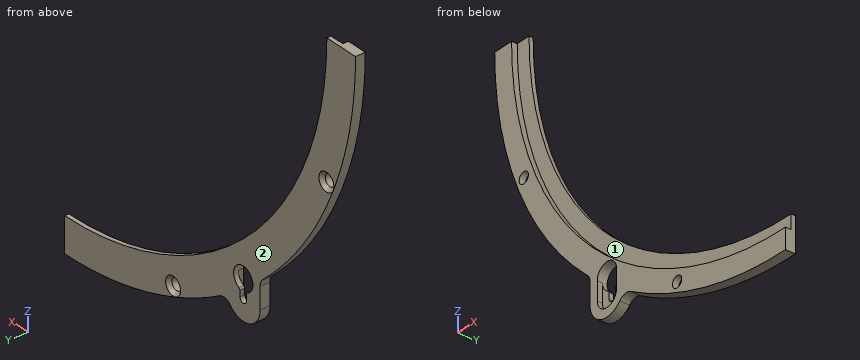
```python
from build123d import *

# Parameters (mm, degrees)
CUT_EXTRUDE2_DEPTH                   = 25.4
F_6_0_204_DIAMETER_HOLE1_D           = 5.499999922
F_6_0_204_DIAMETER_HOLE1_CSINK_D     = 8.89
F_6_0_204_DIAMETER_HOLE1_CSINK_ANGLE = 90
BOSS_EXTRUDE2_REACH                  = 245.998
CUT_EXTRUDE3_DEPTH                   = 244.998078886
CUT_EXTRUDE4_DEPTH                   = 2.5
FILLET1_R                            = 5
FILLET3_R                            = 1


with BuildPart() as part:
    # Sketch1 → Revolve1 (revolve)
    with BuildSketch(Plane.XY, mode=Mode.PRIVATE) as revolve1_sk:
        Polygon((-162.5, 0), (-162.5, 2.75), (-155.5, 2.75), (-155.5, 4.75), (-172.5, 4.75), (-172.5, 0), align=None)
    revolve(revolve1_sk.sketch.rotate(Axis((0, 0, 0), (0, 1, 0)), 270), axis=Axis((0, 0, 0), (0, 1, 0)))

    # Sketch5 → Cut-Extrude2 (cut, symmetric)
    with BuildSketch(Plane(origin=(0, 0, 0), x_dir=(1, 0, 0), z_dir=(0, 1, 0))):
        with BuildLine():
            Line((0, 0), (0, 184.517203458))
            ThreePointArc((0, 184.517203458), (-130.473365811, -130.473365811), (184.517203458, 0))
            Line((184.517203458, 0), (0, 0))
        make_face()
    extrude(amount=CUT_EXTRUDE2_DEPTH, both=True, mode=Mode.SUBTRACT)

    # #6 (0.204) Diameter Hole1 (through all)
    with Locations(Plane(origin=(0, 4.75, 0), x_dir=(1, 0, 0), z_dir=(0, 1, 0))):
        with Locations((155.211761462, 64.290816637), (64.290816637, 155.211761462)):
            CounterSinkHole(F_6_0_204_DIAMETER_HOLE1_D / 2, F_6_0_204_DIAMETER_HOLE1_CSINK_D / 2, counter_sink_angle=F_6_0_204_DIAMETER_HOLE1_CSINK_ANGLE)

    # Boss-Extrude2: up to this face of the body (flat: up to its plane)
    boss_extrude2_end = Plane(part.part.faces().sort_by_distance((111.680104475, 4.75, -111.680104475))[0])
    # Sketch13 → Boss-Extrude2 (add, up to the picked face)
    with BuildSketch(Plane(origin=(0, 0, 0), x_dir=(1, 0, 0), z_dir=(0, 1, 0)), mode=Mode.PRIVATE) as boss_extrude2_sk1:
        with BuildLine():
            Line((115.914175626, 113.837772395), (115.914175626, 140.5528583))
            ThreePointArc((115.914175626, 140.5528583), (105.914175626, 150.5528583), (95.914175626, 140.5528583))
            Line((95.914175626, 140.5528583), (95.914175626, 135.636049675))
            Line((95.914175626, 135.636049675), (115.914175626, 113.837772395))
        make_face()
    boss_extrude2_tool1 = split(extrude(boss_extrude2_sk1.sketch, amount=BOSS_EXTRUDE2_REACH, mode=Mode.PRIVATE), bisect_by=boss_extrude2_end, keep=Keep.BOTH, mode=Mode.PRIVATE)
    add(boss_extrude2_tool1.solids().sort_by(Axis((107.449054, 0, -135.840664), (0, 1, 0)))[0])

    # Sketch8 → Cut-Extrude3 (cut, through all)
    with BuildSketch(Plane.XZ):
        with BuildLine():
            Line((104.009175626, -136.941011973), (104.009175626, -140.5528583))
            ThreePointArc((104.009175626, -140.5528583), (105.914175626, -142.4578583), (107.819175626, -140.5528583))
            Line((107.819175626, -140.5528583), (107.819175626, -136.941011973))
            ThreePointArc((107.819175626, -136.941011973), (105.914175626, -125.8378583), (104.009175626, -136.941011973))
        make_face()
    extrude(amount=-CUT_EXTRUDE3_DEPTH, mode=Mode.SUBTRACT)

    # Sketch9 → Cut-Extrude4 (cut)
    with BuildSketch(Plane.XZ):
        with BuildLine():
            Line((111.629175626, -140.5528583), (111.629175626, -131.5528583))
            ThreePointArc((111.629175626, -131.5528583), (105.914175626, -125.8378583), (100.199175626, -131.5528583))
            Line((100.199175626, -131.5528583), (100.199175626, -140.5528583))
            ThreePointArc((100.199175626, -140.5528583), (105.914175626, -146.2678583), (111.629175626, -140.5528583))
        make_face()
    extrude(amount=-CUT_EXTRUDE4_DEPTH, mode=Mode.SUBTRACT)

    # Fillet1
    fillet1_edges = [part.edges().sort_by_distance(p)[0] for p in [
        (115.914175626, 2.375, -127.750357687),
        (96.256410587, 2.375, -143.146615122),
    ]]
    fillet(fillet1_edges, radius=FILLET1_R)


with BuildPart() as body_2:
    # Mirror1: mirrored copy
    add(part.part.mirror(Plane(origin=(0, 0, 0), x_dir=(0, 0, 1), z_dir=(1, 0, 0))))

    # Fillet3
    fillet3_edges = [body_2.edges().sort_by_distance(p)[0] for p in [
        (-104.009175626, 3.625, -136.941011973),
        (-107.819175626, 3.625, -136.941011973),
    ]]
    fillet(fillet3_edges, radius=FILLET3_R)


solid = body_2.part
```
Could you check a few things on this model? Use its own coordinates, in mm. Face numbers are marked on the shaded views. Round coordinates to 2 decimals unless told otherwise and drop trailing zeros. Loops run counter-clockwise (first coordinate to the right, second up) from the corner with the lowest first, then second, coordinate; pieces in that order, holes last. Notation, with made-up numbers: (-6, -14.5) - (32, -14.5) arc R20 cw to (32, 5.5) - close; hole circle Ø10 at (77, 4.25). An arc over 180 degrees is marked (long way). Answer as CSV lines item,"result".
1. Please list where these lines run through material, in increasing order: line 1 along Y through (x, z) = (-50.5, -151); line 2 along Z through (x, y) = (-101.5, 3.05); line 3 along X through (y, z) = (1.7, -101). Write a range as [from, to].
Filled in:
line 1,"y = [2.75, 4.75]"
line 2,"z = [-149.53, -135.18], [-127.92, -117.8]"
line 3,"x = [-139.84, -127.3]"
2. We'd pull the mould along Y, two halves only. Please class the marked faces 1 and 2: +Y half, -Y half, draft (parallel to the pull), parting line (faces both ways), or undercut.
Filled in:
face 1,"-Y half"
face 2,"+Y half"
3. I want a section at A-A on z = -43.5. List the corners of the cut face in (x, y) for me, then the cut area to 3 significant figures.
Filled in:
outline,"(-166.93, 0) - (-156.57, 0) - (-156.57, 2.75) - (-149.29, 2.75) - (-149.29, 4.75) - (-166.93, 4.75) - close"
area,"63.7 mm^2"
4. I want a section at C-C on y = 1.2. Count the separate pieces of the cut face and the enclosed holes in it, then the cut area to 3 significant figures.
Filled in:
separate pieces,"1"
enclosed holes,"3"
area,"2,630 mm^2"
5. For pin 1 Ø0.8 at (y, z) = (0.5, -137.5) entering from +X; pin 2 Ø1 at (x, y) = (-68.5, 3) entering from -Z; pin 3 Ø0.7 at (y, z) = (3, -139) entering from +X, each with a flat end and sliding along its axis, tell me the tip position at first contact or that it passes through.
Filled in:
pin 1,"stops at x = -85.96"
pin 2,"stops at z = -158.53"
pin 3,"stops at x = -69.01"
6. I want a section at B-B on x = -125. List the corners of the cut face in (y, z) for me, then the cut area to 3 significant figures.
Filled in:
outline,"(0, -118.87) - (4.75, -118.87) - (4.75, -92.49) - (2.75, -92.49) - (2.75, -103.83) - (0, -103.83) - close"
area,"94.1 mm^2"
